from build123d import *

# Parameters (mm, degrees)
F0_W     = 50
F0_H     = 40
F0_R     = 2
F1_DEPTH = 4
F2_R     = 4
F2_R_2   = 2
F3_DEPTH = 2
F5_DEPTH = 25


with BuildPart() as f1:
    # F0 (on Front) → F1 (new body)
    with BuildSketch(Plane.XZ):
        Rectangle(F0_W, F0_H)
        with Locations((-20, -15)):
            Circle(F0_R, mode=Mode.SUBTRACT)
        with Locations((20, -15)):
            Circle(F0_R, mode=Mode.SUBTRACT)
        with Locations((-20, 15)):
            Circle(F0_R, mode=Mode.SUBTRACT)
        with Locations((20, 15)):
            Circle(F0_R, mode=Mode.SUBTRACT)
    extrude(amount=F1_DEPTH)

    # F2 (on face) → F3 (cut)
    with BuildSketch(Plane.XZ.offset(4)):
        with Locations((-20, 15)):
            Circle(F2_R)
        with Locations((-20, 15)):
            Circle(F2_R_2, mode=Mode.SUBTRACT)
        with Locations((20, 15)):
            Circle(F2_R)
        with Locations((20, 15)):
            Circle(F2_R_2, mode=Mode.SUBTRACT)
        with Locations((20, -15)):
            Circle(F2_R)
        with Locations((20, -15)):
            Circle(F2_R_2, mode=Mode.SUBTRACT)
        with Locations((-20, -15)):
            Circle(F2_R)
        with Locations((-20, -15)):
            Circle(F2_R_2, mode=Mode.SUBTRACT)
    extrude(amount=-F3_DEPTH, mode=Mode.SUBTRACT)

    # F4 (on face) → F5 (cut)
    with BuildSketch(Plane.XZ.offset(4)):
        with BuildLine():
            Line((3.000102, 5.749591), (2.953973, 0.156237))
            ThreePointArc((2.953973, 0.156237), (6.025203, -14.197312), (8.999898, 0.176554))
            Line((8.999898, 0.176554), (8.999898, 5.70011))
            ThreePointArc((8.999898, 5.70011), (9, 5.724851), (8.999898, 5.749591))
            ThreePointArc((8.999898, 5.749591), (6, 8.724851), (3.000102, 5.749591))
        make_face()
    extrude(amount=-F5_DEPTH, mode=Mode.SUBTRACT)


solid = f1.part
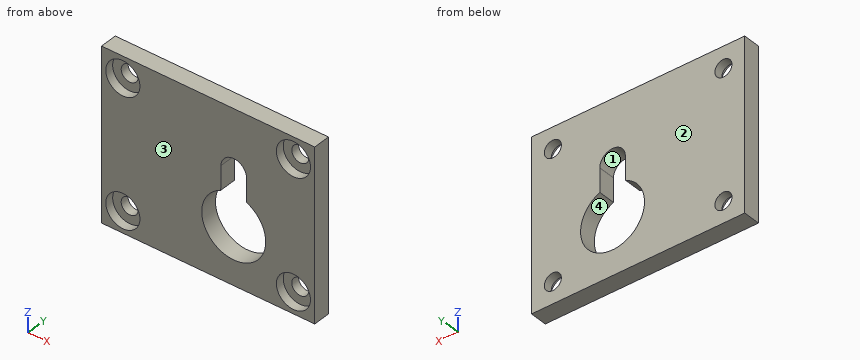
Check sheet for the modelled part. Datum: model origin and axes. Units: mm. Face numbers are marked on the shaded views. A direction names the side the tool comes from. Round coordinates to 2 decimals unless told otherwise and drop trailing zeros. Write each loop counter-clockwise with the first axis right and the second up, starting at its lowest first coordinate (ties: lowest second). Pieces come first, ordered by that corner, then holes. Notation, with made-up numbers: (-28.75, -19.75) - (16.25, -19.75) arc R30 cw to (16.25, 9.25) - close; hole circle Ø8 at (35.5, 59). An arc over 180 degrees is marked (long way). Return JSON: item names as keys, results as strings.
Q1. Cross-section at B-B (x = -20). Record the boundary of the cut face in (y, z), then the cut area to 3 significant figures.
Returned:
{"outline": "(-4, -20) - (0, -20) - (0, -17) - (-2, -17) - (-2, -19) - (-4, -19) - close; (-4, -11) - (-2, -11) - (-2, -13) - (0, -13) - (0, 13) - (-2, 13) - (-2, 11) - (-4, 11) - close; (-4, 19) - (-2, 19) - (-2, 17) - (0, 17) - (0, 20) - (-4, 20) - close", "area": "112 mm²"}
Q2. Draft check along X on the marked faces 3 and 4. Enter one of: released by +X, released by -X, zero draft, split by the parting line, or undercut.
Returned:
{"face 3": "zero draft", "face 4": "undercut"}
Q3. Depth check by flat-ended pin: P1, Ø4, axis at x = -20, z = 14.5, coming from the -Y side. Enter the tip coordinate at first touch or a pass-through.
Returned:
{"P1": "stops at y = -2"}
Q4. Access from +Z, -Z, +X, -X, +Y, -Y to the whole of each face (thin tool, end or side, straight path). Record for the marked faces 1 and 2.
Returned:
{"face 1": "+Y, -Y", "face 2": "+Z, -Z, +X, -X, +Y"}
Q5. Cross-section at A-A (z = 15). Record the boundary of the cut face in (x, y), then the cut area to 3 significant figures.
Returned:
{"outline": "(-25, -4) - (-24, -4) - (-24, -2) - (-22, -2) - (-22, 0) - (-25, 0) - close; (-18, -2) - (-16, -2) - (-16, -4) - (16, -4) - (16, -2) - (18, -2) - (18, 0) - (-18, 0) - close; (22, -2) - (24, -2) - (24, -4) - (25, -4) - (25, 0) - (22, 0) - close", "area": "152 mm²"}
Q6. Cross-section at D-D (y = -0.6). Record the boundary of the cut face in (x, z), then the cut area to 3 significant figures.
Returned:
{"outline": "(-25, -20) - (25, -20) - (25, 20) - (-25, 20) - close; hole circle Ø4 at (-20, -15); hole circle Ø4 at (-20, 15); hole (2.95, 0.16) arc R7.5 ccw (long way) to (9, 0.18) - (9, 5.7) arc R3 ccw to (9, 5.75) arc R3 ccw to (3, 5.75) - close; hole circle Ø4 at (20, -15); hole circle Ø4 at (20, 15)", "area": "1,730 mm²"}
Q7. Cross-section at C-C (x = 6). Record the boundary of the cut face in (y, z), then the cut area to 3 significant figures.
Returned:
{"outline": "(-4, -20) - (0, -20) - (0, -14.2) - (-4, -14.2) - close; (-4, 8.72) - (0, 8.72) - (0, 20) - (-4, 20) - close", "area": "68.3 mm²"}
Q8. Scan lines: L1, parallel to Z at x = -20, y = -3.25; L2, parallel to X at y = -3.55, z = 14.5; L3, parallel to X at y = -0.75, z = -16.5. Record each from-to range of solid material in increasing order. Write a range as from..to.
Returned:
{"L1": "z = -20..-19, -11..11, 19..20", "L2": "x = -25..-23.97, -16.03..16.03, 23.97..25", "L3": "x = -25..-21.32, -18.68..18.68, 21.32..25"}
